Geometry check sheet. Reference: the model listing, model coordinates, mm. A direction names the side the tool comes from. Give positions to 0.01 mm unless a question says otherwise; leave off trailing zeros. Write each loop counter-clockwise with the first axis right and the second up, starting at its lowest first coordinate (ties: lowest second). Pieces come first, ordered by that corner, then holes.
(1) Thickness scan on line 1 along X through (y, z) = (2.5, 6); line 2 along Y through (x, z) = (0, 0.75); line 3 along Z through (x, y) = (-3.75, 4.5). Record the ranges inside material, lowest first.
(2) Cross-section at D-D (x = 4.5). Record the boundary of the cut face in (y, z).
(3) Depth check by flat-ended pin: P1, Ø0.7, axis at x = -10, z = 3.5, coming from the -Y side; P2, Ø4.5, axis at x = 5.5, y = -2, coming from the +Z side; P3, Ø0.7, axis at x = 9.5, z = 3.5, coming from the +Y side; P4, Ø2, axis at y = -1, z = 4.5, coming from the +X side. Enter the tip coordinate at first touch or a pass-through.
(4) Cross-section at B-B (z = 2.25). Record the boundary of the cut face in (x, y), and give its area (3 significant figures).
(5) Tool access check on faces 4 (the flat face through (9.195, 0, 5)), 5 (the flat face through (-9, 6.35, 5)), 6 (the flat face through (-10, 0, 7.874)), 7 (the flat face through (8.306, 0, 5)), 8 (the flat face through (9, -6.35, 5)). Record the directions out of +Z, -Z, +X, -X, +Y, -Y that give a thin tool (end or side, any length) a straight path to the whole face; none if there is none.
(6) Cross-section at A-A (x = 0). Record the boundary of the cut face in (y, z), and give its area (3 significant figures).
(7) Cross-section at C-C (y = 0). Record the boundary of the cut face in (x, z) (3 decimals).
(8) Mould release check, pull along X, two halves, no side actions. Record for faces 1 (the cylindrical face through (3.05, -1.26, 0.75)), 2 (the flat face through (-0.2, 3.5, 0)), 3 (the flat face through (-9.195, 0, 5)): +X half, -X half, draft (parallel to the pull), parting line (faces both ways), or undercut.
```python
from build123d import *

# Parameters (mm, degrees)
F0_W        = 21.59
F0_H        = 15.24
F0_W_2      = 0.889
F0_H_2      = 12.7
F0_R        = 3.302
F1_DEPTH    = 1.524
F2_DEPTH    = 8.89
F3_W        = 12.7
F3_H        = 1.016
F5_DEPTH    = 1.6002
F4_W        = 12.7
F4_H        = 1.016
F6_DEPTH    = 1.6002
F7_T1_DEPTH = 19.2320747894
F8_R        = 1.905


# Not quite as in the source:
# - a fillet or chamfer that OpenCascade refuses, or shapes differently, is made with other operations: its cross-section is extruded or revolved along the edge and cut away or added


with BuildPart() as f1:
    # F0 (on Top) → F1 (new body)
    with BuildSketch(Plane.XY):
        Rectangle(F0_W, F0_H)
        with Locations((-8.7503, 0)):
            Rectangle(F0_W_2, F0_H_2, mode=Mode.SUBTRACT)
        Circle(F0_R, mode=Mode.SUBTRACT)
        with Locations((8.7503, 0)):
            Rectangle(F0_W_2, F0_H_2, mode=Mode.SUBTRACT)
    extrude(amount=F1_DEPTH)

    # F0 (on Top) → F2 (join)
    with BuildSketch(Plane.XY):
        with Locations((-8.7503, 0)):
            Rectangle(F0_W_2, F0_H_2)
        with Locations((8.7503, 0)):
            Rectangle(F0_W_2, F0_H_2)
    extrude(amount=F2_DEPTH)

    # F3 (on face) → F5 (join)
    with BuildSketch(Plane(origin=(-9.1948, 0, 0), x_dir=(0, -1, 0), z_dir=(-1, 0, 0))):
        with Locations((0, 8.382)):
            Rectangle(F3_W, F3_H)
    extrude(amount=F5_DEPTH)

    # F4 (on face) → F6 (join)
    with BuildSketch(Plane.YZ.offset(9.1948)):
        with Locations((0, 8.382)):
            Rectangle(F4_W, F4_H)
    extrude(amount=F6_DEPTH)

    # F7: chamfer of 1.27 on 2 edges, made by hand

    # F7_s2 → F7_t1 (cut)
    with BuildSketch(Plane.XZ.offset(-9.6160373947)):
        Polygon((-10.795, 7.62), (-9.525, 8.89), (-10.795, 8.89), align=None)
        Polygon((10.795, 7.62), (9.525, 8.89), (10.795, 8.89), align=None)
    extrude(amount=F7_T1_DEPTH, mode=Mode.SUBTRACT)

    # F8
    f8_edges = [f1.edges().sort_by_distance(p)[0] for p in [
        (10.795, -7.62, 0.762),
        (10.795, 7.62, 0.762),
        (-10.795, 7.62, 0.762),
        (-10.795, -7.62, 0.762),
    ]]
    fillet(f8_edges, radius=F8_R)


solid = f1.part
```
Reply:
1. line 1: x = -9.19 to -8.31, 8.31 to 9.19
1. line 2: y = -7.62 to -3.3, 3.3 to 7.62
1. line 3: z = 0 to 1.52
2. outline: (-7.62, 0) - (7.62, 0) - (7.62, 1.52) - (-7.62, 1.52) - close
3. P1: passes through
3. P2: stops at z = 1.52
3. P3: stops at y = 6.35
3. P4: stops at x = 9.19
4. outline: (-9.19, -6.35) - (-8.31, -6.35) - (-8.31, 6.35) - (-9.19, 6.35) - close; (8.31, -6.35) - (9.19, -6.35) - (9.19, 6.35) - (8.31, 6.35) - close
4. area: 22.6 mm2
5. face 4: +X, +Y, -Y
5. face 5: +Z, +X, -X, +Y
5. face 6: -X, +Y, -Y
5. face 7: +Z, +Y, -Y
5. face 8: +Z, +X, -X, -Y
6. outline: (-7.62, 0) - (-3.3, 0) - (-3.3, 1.52) - (-7.62, 1.52) - close; (3.3, 0) - (7.62, 0) - (7.62, 1.52) - (3.3, 1.52) - close
6. area: 13.2 mm2
7. outline: (-10.795, 0) - (-3.302, 0) - (-3.302, 1.524) - (-8.306, 1.524) - (-8.306, 8.89) - (-9.525, 8.89) - (-10.541, 7.874) - (-9.195, 7.874) - (-9.195, 1.524) - (-10.795, 1.524) - close; (3.302, 0) - (10.795, 0) - (10.795, 1.524) - (9.195, 1.524) - (9.195, 7.874) - (10.541, 7.874) - (9.525, 8.89) - (8.306, 8.89) - (8.306, 1.524) - (3.302, 1.524) - close
8. face 1: undercut
8. face 2: draft
8. face 3: -X half
